Input: part model. Units: mm. Frame: model coordinates. Face numbers are marked on the shaded views. Round coordinates to 2 decimals unless told otherwise and drop trailing zeros. Loops run counter-clockwise (first coordinate to the right, second up) from the corner with the lowest first, then second, coordinate; pieces in that order, holes last.
(1) Cut plane C-C, the plane z = 7.25. Output: boundary loops of the cut face in (x, y), and give its area (3 significant figures).
(2) Draft query along Y for the marked faces 1, 2 and 3. Return one class per face: released by +Y, released by -Y, zero draft, split by the parting line, or undercut.
(3) Cut plane B-B, the plane x = 7.5. Output: boundary loops of the cut face in (y, z), and give its area (3 significant figures).
(4) First-contact query: pin 1 Ø3 at (x, y) = (-7.5, 0) entering from +Z. Flat tip, straight axial feed; report the tip coordinate or a pass-through.
(5) Cut plane D-D, the plane y = -4. Output: boundary loops of the cut face in (x, z), and give its area (3 significant figures).
(6) Line query: line 1 (Y direction, x = -7.5, z = 6.25); line 2 (Y direction, x = 9, z = 7.5); line 3 (X direction, y = -1, z = 7). Output: solid intervals per line, ascending.
(7) Cut plane A-A, the plane y = 0. Output: boundary loops of the cut face in (x, z).
from build123d import *

# Parameters (mm, degrees)
SKETCH_1_W          = 30
SKETCH_1_H          = 10
EXTRUDE_1_DEPTH     = 8
FILLET_1_R          = 2
SKETCH_3_R          = 1.65
CUT_EXTRUDE_1_DEPTH = 9


with BuildPart() as part:
    # 草图1 → 凸台-拉伸1 (new body)
    with BuildSketch(Plane.XY):
        Rectangle(SKETCH_1_W, SKETCH_1_H)
    extrude(amount=EXTRUDE_1_DEPTH)

    # 圆角1
    fillet_1_edges = [part.edges().sort_by_distance(p)[0] for p in [
        (15, -5, 4),
        (-15, -5, 4),
        (-15, 5, 4),
        (15, 5, 4),
    ]]
    fillet(fillet_1_edges, radius=FILLET_1_R)

    # 草图3 → 切除-拉伸1 (cut, through all)
    with BuildSketch(Plane(origin=(0, 0, 0), x_dir=(-1, 0, 0), z_dir=(0, 0, -1))):
        with Locations((-7.5, 0)):
            Circle(SKETCH_3_R)
        with Locations((7.5, 0)):
            Circle(SKETCH_3_R)
    extrude(amount=-CUT_EXTRUDE_1_DEPTH, mode=Mode.SUBTRACT)


solid = part.part
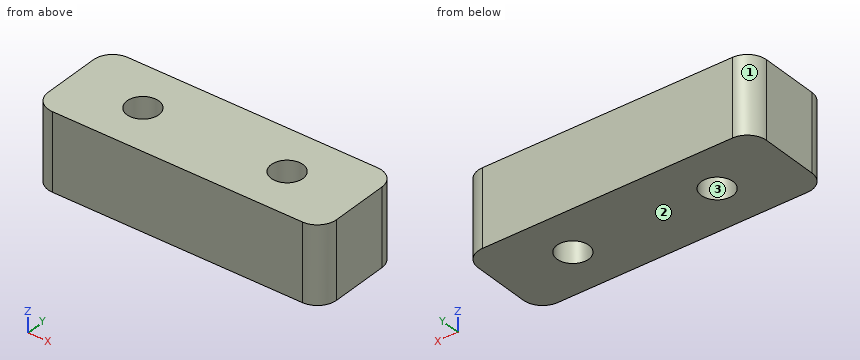
Reported:
1. outline: (-15, -3) arc R2 ccw to (-13, -5) - (13, -5) arc R2 ccw to (15, -3) - (15, 3) arc R2 ccw to (13, 5) - (-13, 5) arc R2 ccw to (-15, 3) - close; hole circle Ø3.3 at (-7.5, 0); hole circle Ø3.3 at (7.5, 0)
1. area: 279 mm2
2. face 1: released by +Y
2. face 2: zero draft
2. face 3: undercut
3. outline: (-5, 0) - (-1.65, 0) - (-1.65, 8) - (-5, 8) - close; (1.65, 0) - (5, 0) - (5, 8) - (1.65, 8) - close
3. area: 53.6 mm2
4. pin 1: passes through
5. outline: (-14.73, 0) - (14.73, 0) - (14.73, 8) - (-14.73, 8) - close
5. area: 236 mm2
6. line 1: y = -5 to -1.65, 1.65 to 5
6. line 2: y = -5 to -0.69, 0.69 to 5
6. line 3: x = -15 to -8.81, -6.19 to 6.19, 8.81 to 15
7. outline: (-15, 0) - (-9.15, 0) - (-9.15, 8) - (-15, 8) - close; (-5.85, 0) - (5.85, 0) - (5.85, 8) - (-5.85, 8) - close; (9.15, 0) - (15, 0) - (15, 8) - (9.15, 8) - close
